Could you check a few things on this model? Use its own coordinates, in mm. A direction names the side the tool comes from. Give positions to 0.01 mm unless a question says otherwise; leave off trailing zeros. Use one line per item in the form item = value.
```python
from build123d import *

# Parameters (mm, degrees)
SKETCH1_W                                           = 384
SKETCH1_H                                           = 110
EXTRUDE2_DEPTH                                      = 8
CBORE_FOR_M5_HEX_SOCKET_HEAD_CAP_SCREW1_D           = 5.5
CBORE_FOR_M5_HEX_SOCKET_HEAD_CAP_SCREW1_CBORE_D     = 10
CBORE_FOR_M5_HEX_SOCKET_HEAD_CAP_SCREW1_CBORE_DEPTH = 5.4


with BuildPart() as part:
    # Sketch1 → Extrude2 (new body)
    with BuildSketch(Plane.XY):
        with Locations((192, 55)):
            Rectangle(SKETCH1_W, SKETCH1_H)
    extrude(amount=EXTRUDE2_DEPTH)

    # CBORE for M5 Hex Socket Head Cap Screw1 (through all)
    with Locations(Plane(origin=(362, 95, 0), x_dir=(-1, 0, 0), z_dir=(0, 0, -1))):
        with Locations((0, 0), (340, 0), (340, -80), (0, -80)):
            CounterBoreHole(CBORE_FOR_M5_HEX_SOCKET_HEAD_CAP_SCREW1_D / 2, CBORE_FOR_M5_HEX_SOCKET_HEAD_CAP_SCREW1_CBORE_D / 2, CBORE_FOR_M5_HEX_SOCKET_HEAD_CAP_SCREW1_CBORE_DEPTH)


solid = part.part
```
1. If we mould it in two halves opening along X, with no side actions, what happens to faces 1 (the face through (0, 54, 4)), 2 (the face through (189, 56, 0)), 3 (the face through (357.381, 13.085, 2.662))? For each: pulls with the +X half, pulls with the -X half, needs draft (parallel to the pull), parting line crosses it, or undercut.
Response values:
face_1 = pulls with the -X half
face_2 = needs draft
face_3 = undercut
2. For pin 1 (3 mm diameter, centred on x = 22.5, y = 13.5, fed in from -Z), with a flat end and sliding along its axis, tell me the tip position at first contact or that it passes through.
Response values:
pin_1 = 5.4
3. If I drill on line 1 (Y direction, x = 362, z = 6.15); line 2 (Y direction, x = 22, z = 4.3); line 3 (X direction, y = 18.5, z = 2), over which ranges is the centre line in solid material (lowest first)? Write a range as from..to.
Response values:
line_1 = 0..12.25, 17.75..92.25, 97.75..110
line_2 = 0..10, 20..90, 100..110
line_3 = 0..18.43, 25.57..358.43, 365.57..384
4. Which directions (+Z, -Z, +X, -X, +Y, -Y) give clear straight access to the entire face, cutting with the end or side of a thin tool? Please do faces 4 (the face through (359.8, 92.8, 5.4)), 5 (the face through (189, 0, 4)).
Response values:
face_4 = -Z
face_5 = +Z, -Z, +X, -X, -Y
